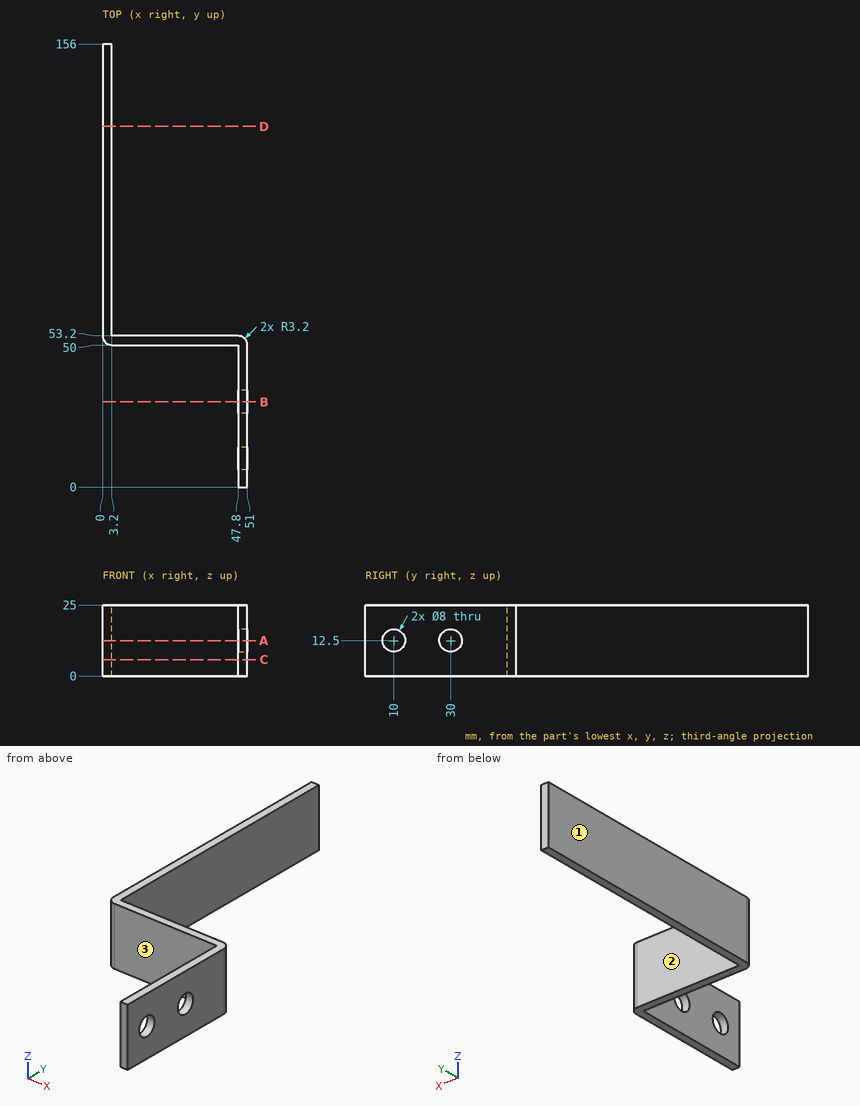
Answer from the drawing. Dimensions are ordinates in mm from the lowest x, y and z of the part. A direction names the side the tool comes from. Give positions to 0.01 mm unless a question says otherwise; leave off trailing zeros. Loops run counter-clockwise (first coordinate to the right, second up) from the corner with the lowest first, then second, coordinate; pieces in that order, holes last.
Item 1: A cutting plane is placed at C-C (z = 5.75). Give the vertices of the cut face in (x, y), then the cut area to 3 significant figures.
Derived:
outline: (0, 53.2) arc R3.2 ccw to (3.2, 50) - (47.8, 50) - (47.8, 0) - (51, 0) - (51, 50) arc R3.2 ccw to (47.8, 53.2) - (3.2, 53.2) - (3.2, 156) - (0, 156) - close
area: 648 mm2
Item 2: Find the intervals of material crossed by line 1 along Z through (x, y) = (50, 10); line 2 along Y through (x, z) = (49.6, 12.5); line 3 along X through (y, z) = (105.5, 9.25), in increasing order.
Derived:
line 1: z = 0 to 8.5, 16.5 to 25
line 2: y = 0 to 6, 14 to 26, 34 to 52.65
line 3: x = 0 to 3.2
Item 3: Each of these flat-tipped pins is pushed along its axis until it touches: pin 1 Ø1 at (y, z) = (75, 21) entering from +X; pin 2 Ø10.5 at (y, z) = (10, 12.5) entering from +X; pin 3 Ø1.5 at (x, z) = (34.5, 9.5) entering from -Y. Where does it stop, or does it pass through?
Derived:
pin 1: stops at x = 3.2
pin 2: stops at x = 51
pin 3: stops at y = 50
Item 4: A cutting plane is placed at A-A (z = 12.5). Give the vertices of the cut face in (x, y).
Derived:
outline: (0, 53.2) arc R3.2 ccw to (3.2, 50) - (47.8, 50) - (47.8, 34) - (51, 34) - (51, 50) arc R3.2 ccw to (47.8, 53.2) - (3.2, 53.2) - (3.2, 156) - (0, 156) - close; (47.8, 0) - (51, 0) - (51, 6) - (47.8, 6) - close; (47.8, 14) - (51, 14) - (51, 26) - (47.8, 26) - close
Item 5: A cutting plane is placed at D-D (y = 127). Give the vertices of the cut face in (x, z).
Derived:
outline: (0, 0) - (3.2, 0) - (3.2, 25) - (0, 25) - close
Item 6: A cutting plane is placed at B-B (y = 30). Give the vertices of the cut face in (x, z).
Derived:
outline: (47.8, 0) - (51, 0) - (51, 8.5) - (47.8, 8.5) - close; (47.8, 16.5) - (51, 16.5) - (51, 25) - (47.8, 25) - close
Item 7: A tool of negligible diameter and unlimited length cuts with its end or side. For the marked faces 1, 2 and 3, from which of +Z, -Z, +X, -X, +Y, -Y can it reach the whole face along a straight path? Write none if from no direction.
Derived:
face 1: +Z, -Z, -X, +Y, -Y
face 2: +Z, -Z, +X, +Y
face 3: +Z, -Z, -X, -Y
